from build123d import *

# Parameters (mm, degrees)
F0_R     = 5
F1_DEPTH = 4
F2_R     = 2.5
F3_DEPTH = 10
F4_R     = 3.5
F5_DEPTH = 2
F6_R     = 1
F7_DEPTH = 5
F8_SIZE  = 0.2


with BuildPart() as f1:
    # F0 (on Top) → F1 (new body)
    with BuildSketch(Plane.XY):
        Circle(F0_R)
    extrude(amount=F1_DEPTH)

    # F2 (on face) → F3 (join)
    with BuildSketch(Plane.XY.offset(4)):
        Circle(F2_R)
    extrude(amount=F3_DEPTH)

    # F4 (on face) → F5 (join)
    with BuildSketch(Plane.XY.offset(14)):
        Circle(F4_R)
    extrude(amount=F5_DEPTH)

    # F6 (on face) → F7 (join)
    with BuildSketch(Plane.XY.offset(16)):
        Circle(F6_R)
    extrude(amount=F7_DEPTH)

    # F8
    f8_edges = [f1.edges().sort_by_distance(p)[0] for p in [
        (-1, 0, 21),
        (-3.5, 0, 16),
        (-3.5, 0, 14),
    ]]
    chamfer(f8_edges, length=F8_SIZE)


solid = f1.part
Work out the finished part from the listing and answer in its coordinate system (mm). A direction names the side the tool comes from. Give positions to 0.01 mm unless a question says otherwise; leave off trailing zeros. Order: outer loops, then holes, each group sorted by start corner. A loop starts at its lowest first (then second) coordinate and runs counter-clockwise, first axis right, second up. Notation, with made-up numbers: (76, 28.5) - (113, 28.5) arc R9 ccw to (113, 44.5) - close; hole circle Ø3 at (7.5, 46.5). An arc over 180 degrees is marked (long way). Answer as CSV lines item,"result". Start each with the question number.
Q1. Find the intervals of material crossed by L1, parallel to Z at x = -1, y = 2.25; L2, parallel to Z at x = 2, y = 3; L3, parallel to Z at x = -1.5, y = 3, in increasing order. Write a range as [from, to].
Q2. The part is cut by section D-D (x = 4). Write down the section's boundary in (y, z), then the cut area to 3 significant figures.
Q3. The part is cut by section A-A (x = 0). Write down the section's boundary in (y, z).
Q4. For faces 1 (the face through (3.233, -1.341, 14.989)), 2 (the face through (2, -2, 4)), 3 (the face through (-1.08, -4.88, 1.97)), determine the directions among +Z, -Z, +X, -X, +Y, -Y from which every point of the face is accessible in a straight line to the end or side of a thin tool.
Q5. The part is cut by section C-C (z = 12.25). Write down the section's boundary in (x, y), then the cut area to 3 significant figures.
Q6. Given pin 1 Ø3 at (x, y) = (-0.5, -2) entering from -Z; pin 2 Ø6 at (x, z) = (3.5, 8.5) entering from +Y; pin 3 Ø1 at (x, z) = (-2, 18) entering from -Y; pin 4 Ø6 at (x, z) = (-2.5, 7.5) entering from -Y, each flat-ended and moving along its own axis, determine where each tip first touches the part or whether it passes through.
Check result:
1,L1,"z = [0, 16]"
1,L2,"z = [0, 4]"
1,L3,"z = [0, 4], [14.05, 15.95]"
2,outline,"(-3, 0) - (3, 0) - (3, 4) - (-3, 4) - close"
2,area,"24.0 mm²"
3,outline,"(-5, 0) - (5, 0) - (5, 4) - (2.5, 4) - (2.5, 14) - (3.3, 14) - (3.5, 14.2) - (3.5, 15.8) - (3.3, 16) - (1, 16) - (1, 20.8) - (0.8, 21) - (-0.8, 21) - (-1, 20.8) - (-1, 16) - (-3.3, 16) - (-3.5, 15.8) - (-3.5, 14.2) - (-3.3, 14) - (-2.5, 14) - (-2.5, 4) - (-5, 4) - close"
4,face 1,"+Z"
4,face 2,"none"
4,face 3,"+Z, -Z"
5,outline,"circle Ø5 at (0, 0)"
5,area,"19.6 mm²"
6,pin 1,"stops at z = 0"
6,pin 2,"stops at y = 2.45"
6,pin 3,"passes through"
6,pin 4,"stops at y = -2.5"
